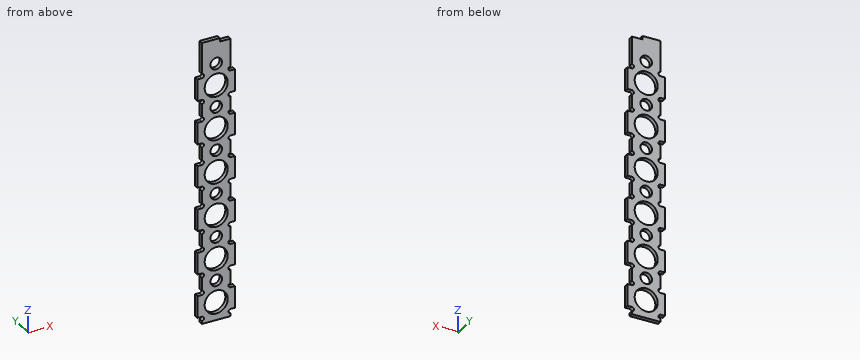
from build123d import *

# Parameters (mm, degrees)
SKETCH_1_W          = 20
SKETCH_1_H          = 194.9
EXTRUDE_1_DEPTH     = 3
SKETCH_2_W          = 7.5
SKETCH_2_H          = 2.9
CUT_EXTRUDE_1_DEPTH = 196.946446765
SKETCH_3_W          = 15
SKETCH_3_H          = 3
EXTRUDE_3_DEPTH     = 3
SKETCH_4_R          = 8
CUT_EXTRUDE_2_DEPTH = 197.275342313
SKETCH_5_R          = 4
CUT_EXTRUDE_3_DEPTH = 197.275342313
SKETCH_6_W          = 12.5
SKETCH_6_H          = 0.5
CUT_EXTRUDE_4_DEPTH = 197.275342313
SKETCH_7_R          = 1.5
CUT_EXTRUDE_5_DEPTH = 10


with BuildPart() as part:
    # 草图1 → 凸台-拉伸1 (new body)
    with BuildSketch(Plane(origin=(0, 0, 0), x_dir=(1, 0, 0), z_dir=(0, 1, 0))):
        with Locations((10, 97.45)):
            Rectangle(SKETCH_1_W, SKETCH_1_H)
    extrude(amount=EXTRUDE_1_DEPTH)

    # 草图2 → 切除-拉伸1 (cut, through all)
    with BuildSketch(Plane(origin=(0, 3, 0), x_dir=(1, 0, 0), z_dir=(0, 1, 0))):
        with Locations((16.25, 1.45)):
            Rectangle(SKETCH_2_W, SKETCH_2_H)
    extrude(amount=-CUT_EXTRUDE_1_DEPTH, mode=Mode.SUBTRACT)

    # 草图3 → 凸台-拉伸3 (add)
    with BuildSketch(Plane.ZY):
        with Locations((-182.4, 1.5)):
            Rectangle(SKETCH_3_W, SKETCH_3_H)
        with Locations((-152.4, 1.5)):
            Rectangle(SKETCH_3_W, SKETCH_3_H)
        with Locations((-122.4, 1.5)):
            Rectangle(SKETCH_3_W, SKETCH_3_H)
        with Locations((-92.4, 1.5)):
            Rectangle(SKETCH_3_W, SKETCH_3_H)
        with Locations((-62.4, 1.5)):
            Rectangle(SKETCH_3_W, SKETCH_3_H)
        with Locations((-32.4, 1.5)):
            Rectangle(SKETCH_3_W, SKETCH_3_H)
    extrude_3 = extrude(amount=EXTRUDE_3_DEPTH)

    # 镜向1: 凸台-拉伸3 across plane
    add(extrude_3.mirror(Plane.ZY.offset(-10)))

    # 草图4 → 切除-拉伸2 (cut, through all)
    with BuildSketch(Plane(origin=(0, 3, 0), x_dir=(1, 0, 0), z_dir=(0, 1, 0))):
        with Locations(Location((10, 182.4, 0), (0, 0, 270))):
            Circle(SKETCH_4_R)
        with Locations(Location((10, 152.4, 0), (0, 0, 270))):
            Circle(SKETCH_4_R)
        with Locations(Location((10, 122.4, 0), (0, 0, 270))):
            Circle(SKETCH_4_R)
        with Locations(Location((10, 92.4, 0), (0, 0, 270))):
            Circle(SKETCH_4_R)
        with Locations(Location((10, 62.4, 0), (0, 0, 270))):
            Circle(SKETCH_4_R)
        with Locations(Location((10, 32.4, 0), (0, 0, 270))):
            Circle(SKETCH_4_R)
    extrude(amount=-CUT_EXTRUDE_2_DEPTH, mode=Mode.SUBTRACT)

    # 草图5 → 切除-拉伸3 (cut, through all)
    with BuildSketch(Plane(origin=(0, 3, 0), x_dir=(1, 0, 0), z_dir=(0, 1, 0))):
        with Locations(Location((10, 167.4, 0), (0, 0, 270))):
            Circle(SKETCH_5_R)
        with Locations(Location((10, 137.4, 0), (0, 0, 270))):
            Circle(SKETCH_5_R)
        with Locations(Location((10, 107.4, 0), (0, 0, 270))):
            Circle(SKETCH_5_R)
        with Locations(Location((10, 77.4, 0), (0, 0, 270))):
            Circle(SKETCH_5_R)
        with Locations(Location((10, 47.4, 0), (0, 0, 270))):
            Circle(SKETCH_5_R)
        with Locations(Location((10, 17.4, 0), (0, 0, 270))):
            Circle(SKETCH_5_R)
    extrude(amount=-CUT_EXTRUDE_3_DEPTH, mode=Mode.SUBTRACT)

    # 草图6 → 切除-拉伸4 (cut, through all)
    with BuildSketch(Plane(origin=(0, 3, 0), x_dir=(1, 0, 0), z_dir=(0, 1, 0))):
        with Locations((6.25, 0.25)):
            Rectangle(SKETCH_6_W, SKETCH_6_H)
    extrude(amount=-CUT_EXTRUDE_4_DEPTH, mode=Mode.SUBTRACT)

    # 草图7 → 切除-拉伸5 (cut)
    with BuildSketch(Plane.XZ):
        with Locations((0, -23.4)):
            Circle(SKETCH_7_R)
        with Locations((0, -41.4)):
            Circle(SKETCH_7_R)
        with Locations((0, -53.4)):
            Circle(SKETCH_7_R)
        with Locations((0, -71.4)):
            Circle(SKETCH_7_R)
        with Locations((0, -83.4)):
            Circle(SKETCH_7_R)
        with Locations((0, -101.4)):
            Circle(SKETCH_7_R)
        with Locations((0, -113.4)):
            Circle(SKETCH_7_R)
        with Locations((0, -131.4)):
            Circle(SKETCH_7_R)
        with Locations((0, -143.4)):
            Circle(SKETCH_7_R)
        with Locations((0, -161.4)):
            Circle(SKETCH_7_R)
        with Locations((0, -173.4)):
            Circle(SKETCH_7_R)
        with Locations((0, -191.4)):
            Circle(SKETCH_7_R)
        with Locations((20, -191.4)):
            Circle(SKETCH_7_R)
        with Locations((20, -173.4)):
            Circle(SKETCH_7_R)
        with Locations((20, -161.4)):
            Circle(SKETCH_7_R)
        with Locations((20, -143.4)):
            Circle(SKETCH_7_R)
        with Locations((20, -131.4)):
            Circle(SKETCH_7_R)
        with Locations((20, -113.4)):
            Circle(SKETCH_7_R)
        with Locations((20, -101.4)):
            Circle(SKETCH_7_R)
        with Locations((20, -83.4)):
            Circle(SKETCH_7_R)
        with Locations((20, -71.4)):
            Circle(SKETCH_7_R)
        with Locations((20, -53.4)):
            Circle(SKETCH_7_R)
        with Locations((20, -41.4)):
            Circle(SKETCH_7_R)
        with Locations((20, -23.4)):
            Circle(SKETCH_7_R)
    extrude(amount=-CUT_EXTRUDE_5_DEPTH, mode=Mode.SUBTRACT)


solid = part.part
Could you check a few things on this model? Use its own coordinates, in mm. Give positions to 0.01 mm unless a question says otherwise; leave off trailing zeros. Order: outer loops, then holes, each group sorted by start corner. A loop starts at its lowest first (then second) coordinate and runs counter-clockwise, first axis right, second up. Notation, with made-up numbers: (73, -13) -> (80, -13) arc R22 cw to (80, 22) -> close; hole circle Ø1 at (18, -16). An arc over 180 degrees is marked (long way). Answer in a Markdown table with one row per item. Add a question column.
Item 1: Imagine slicing it at C-C (z = -49.5). List the corners of the cut face in (x, y) for me.
Item 2: Please list where these lines run through material, in increasing order: probe 1 along Z at (x, y) = (22.25, 1.45); probe 2 along X at (y, z) = (2.2, -77.4); probe 3 along X at (y, z) = (1, -62.4).
Item 3: Imagine slicing it at B-B (y = 2.2). Count the separate pieces of the cut face and the enclosed holes in it, and give its area (3 significant figures).
Item 4: I'm going to push flat-ended pins straight in: P1, Ø1.5, axis at y = 1, z = -169, coming from the -X side; P2, Ø1.5, axis at y = 1, z = -163.5, coming from the +X side; P3, Ø5, axis at x = 10, z = -167.4, coming from the +Y side. Where does each tip first touch, or does it pass through?
Item 5: Imagine slicing it at A-A (z = -77.4). List the corners of the cut face in (x, y) for me.
Result:
| question | item | result |
|---|---|---|
| 1 | outline | (0, 0) -> (6.6, 0) -> (6.6, 3) -> (0, 3) -> close; (13.4, 0) -> (20, 0) -> (20, 3) -> (13.4, 3) -> close |
| 2 | probe 1 | -189.9 to -174.9, -159.9 to -144.9, -129.9 to -114.9, -99.9 to -84.9, -69.9 to -54.9, -39.9 to -24.9 |
| 2 | probe 2 | 0 to 6, 14 to 20 |
| 2 | probe 3 | -3 to 2, 18 to 23 |
| 3 | separate pieces | 1 |
| 3 | enclosed holes | 12 |
| 3 | area | 2,820 mm2 |
| 4 | P1 | x = 0 |
| 4 | P2 | x = 20 |
| 4 | P3 | through |
| 5 | outline | (0, 0) -> (6, 0) -> (6, 3) -> (0, 3) -> close; (14, 0) -> (20, 0) -> (20, 3) -> (14, 3) -> close |
